```python
from build123d import *

# Parameters (mm, degrees)
SZKIC1_W                    = 220
SZKIC1_H                    = 108
DODANIE_WYCI_GNI_CIE1_DEPTH = 62
SZKIC2_W                    = 24.7
SZKIC2_H                    = 20
SZKIC2_W_2                  = 50
SZKIC2_H_2                  = 50
DODANIE_WYCI_GNI_CIE2_DEPTH = 0.5


with BuildPart() as part:
    # Szkic1 → Dodanie-wyciągnięcie1 (new body)
    with BuildSketch(Plane(origin=(0, 0, 0), x_dir=(1, 0, 0), z_dir=(0, 1, 0))):
        Rectangle(SZKIC1_W, SZKIC1_H)
    extrude(amount=DODANIE_WYCI_GNI_CIE1_DEPTH)

    # Szkic2 → Dodanie-wyciągnięcie2 (add)
    with BuildSketch(Plane.ZY.offset(110)):
        with Locations((-36.65, 47)):
            Rectangle(SZKIC2_W, SZKIC2_H)
        with Locations((22, 31)):
            Rectangle(SZKIC2_W_2, SZKIC2_H_2)
    extrude(amount=DODANIE_WYCI_GNI_CIE2_DEPTH)


solid = part.part
```
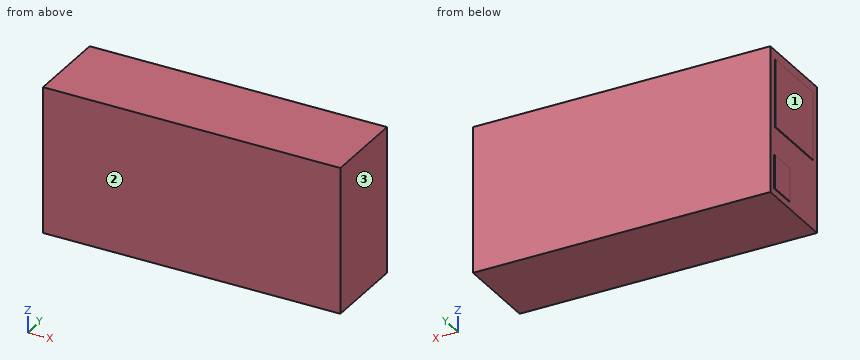
Source: CAD feature listing. Evaluate the final solid. Frame: model axes, mm. Face numbers are marked on the shaded views. Round coordinates to 2 decimals unless told otherwise and drop trailing zeros. One line per item, written item: value. Start each with the question number.
Q1. Material intervals for probe 1 along X at (y, z) = (34, -28), sorted ascending.
Q2. Pin query (flat end, axial travel): pin 1 (0.6 mm diameter, centred on x = -110.5, z = -30.5, fed in from -Y); pin 2 (0.6 mm diameter, centred on x = -110.5, y = 34.5, fed in from +Z); pin 3 (3 mm diameter, centred on y = 36, z = -14.5, fed in from -X). Return the tip coordinate at first contact, or that it passes through.
Q3. Draft query along X for the marked faces 1, 2 and 3. Return one class per face: pulls with the +X half, pulls with the -X half, needs draft (parallel to the pull), parting line crosses it, or undercut.
Findings below:
1. probe 1: -110 to 110
2. pin 1: y = 37
2. pin 2: z = 47
2. pin 3: x = -110
3. face 1: pulls with the -X half
3. face 2: needs draft
3. face 3: pulls with the +X half
